Can you work these out from the drawing? Everything is in mm from the part's minimum corner. Give positions to 0.01 mm unless a question says otherwise; leave off trailing zeros. Write each loop counter-clockwise with the first axis right and the second up, starting at its lowest first coordinate (ties: lowest second). Pieces come first, ordered by that corner, then holes. Notation, with made-up numbers: (-32.75, -32.75) -> (-0.75, -32.75) arc R19 cw to (-0.75, -3.75) -> close; hole circle Ø8 at (42.5, -29). An arc over 180 degrees is marked (long way). Return JSON: item names as keys, results as strings.
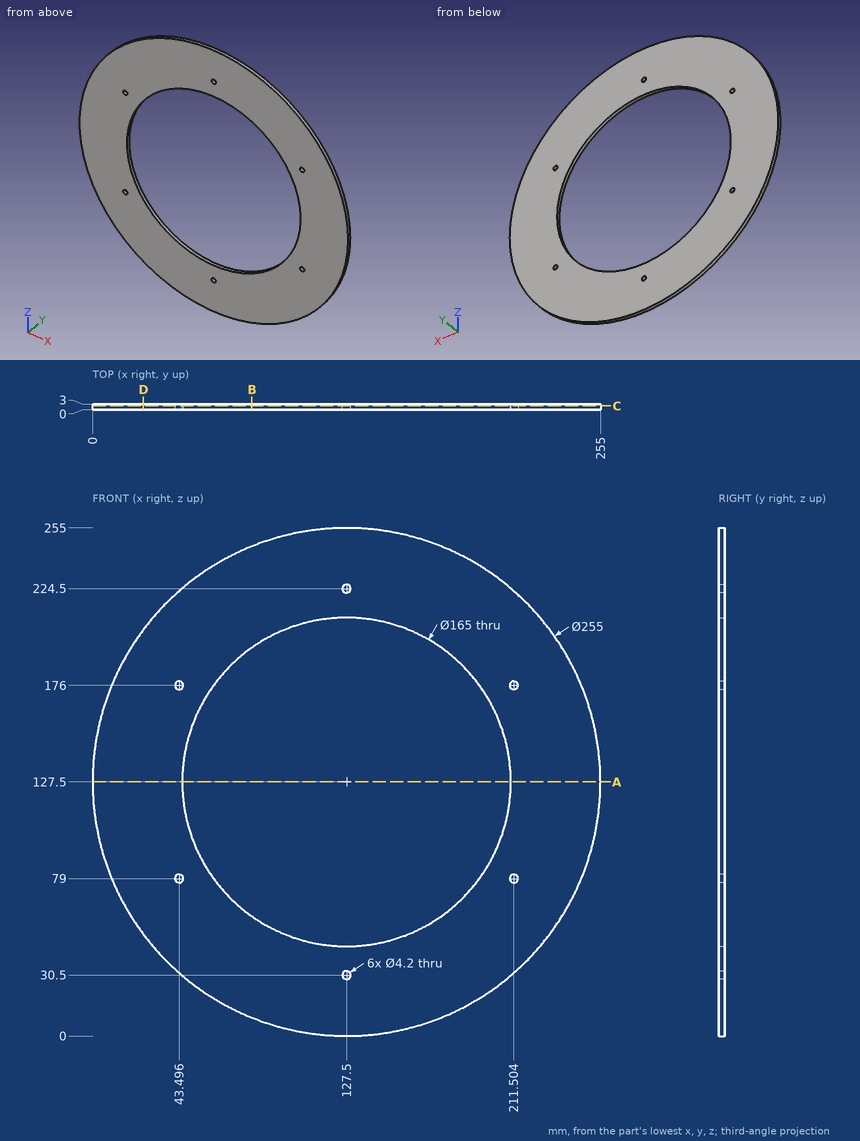
1. Suppose I cut it at D-D, the plane x = 25.5. List the corners of the cut face in (y, z) for me.
Taken from the geometry:
{"outline": "(0, 51) -> (3, 51) -> (3, 204) -> (0, 204) -> close"}
2. Suppose I cut it at A-A, the plane z = 127.5. List the corners of the cut face in (x, y) for me.
Taken from the geometry:
{"outline": "(0, 0) -> (45, 0) -> (45, 3) -> (0, 3) -> close; (210, 0) -> (255, 0) -> (255, 3) -> (210, 3) -> close"}
3. Suppose I cut it at C-C, the plane y = 2. List the corners of the cut face in (x, z) for me (1 decimal).
Taken from the geometry:
{"outline": "circle Ø255 at (127.5, 127.5); hole circle Ø4.2 at (43.5, 79); hole circle Ø4.2 at (43.5, 176); hole circle Ø165 at (127.5, 127.5); hole circle Ø4.2 at (127.5, 30.5); hole circle Ø4.2 at (127.5, 224.5); hole circle Ø4.2 at (211.5, 79); hole circle Ø4.2 at (211.5, 176)"}
4. For pin 1 Ø1.5 at (y, z) = (2.5, 45) entering from +X; pin 2 Ø1 at (y, z) = (1.5, 51.5) entering from +X; pin 3 Ø4 at (x, z) = (127.5, 30.5) entering from +Y; pin 4 Ø1 at (x, y) = (137.5, 2) entering from +Z (1 decimal), each with a flat end and sliding along its axis, tell me the tip position at first contact or that it passes through.
Taken from the geometry:
{"pin 1": "stops at x = 225.34", "pin 2": "stops at x = 230.24", "pin 3": "passes through", "pin 4": "stops at z = 254.6"}
5. If I drill on line 1 (Z direction, x = 127.5, y = 1.05); line 2 (Z direction, x = 132, y = 1.3); line 3 (Z direction, x = 96.5, y = 1.25) (1 decimal), over which ranges is the centre line in solid material (lowest first)? Write a range as [from, to].
Taken from the geometry:
{"line 1": "z = [0, 28.4], [32.6, 45], [210, 222.4], [226.6, 255]", "line 2": "z = [0.08, 45.12], [209.88, 254.92]", "line 3": "z = [3.8, 51], [204, 251.2]"}
6. Suppose I cut it at B-B, the plane x = 80. List the corners of the cut face in (y, z) for me, and give its area (3 significant figures).
Taken from the geometry:
{"outline": "(0, 9.18) -> (3, 9.18) -> (3, 60.05) -> (0, 60.05) -> close; (0, 194.95) -> (3, 194.95) -> (3, 245.82) -> (0, 245.82) -> close", "area": "305 mm²"}
